Design review of the part built by this model. Coordinates are the model's own, in mm. A direction names the side the tool comes from. Coordinates: 2 decimals unless noted, no trailing zeros. Write each loop counter-clockwise with the first axis right and the second up, starting at its lowest first coordinate (ties: lowest second). Pieces come first, ordered by that corner, then holes.
```python
from build123d import *

# Parameters (mm, degrees)
SKETCH1_W           = 7
SKETCH1_H           = 7
BOSS_EXTRUDE1_DEPTH = 5
SKETCH4_R           = 1.65
CUT_EXTRUDE4_DEPTH  = 4
SKETCH6_R           = 1.65
CUT_EXTRUDE6_DEPTH  = 4
SKETCH6_4_R         = 1.65
BOSS_EXTRUDE2_DEPTH = 1.48


with BuildPart() as part:
    # Sketch1 → Boss-Extrude1 (new body)
    with BuildSketch(Plane(origin=(0, 0, 0), x_dir=(1, 0, 0), z_dir=(0, 1, 0))):
        with Locations((-0.67779661, -2.128287226)):
            Rectangle(SKETCH1_W, SKETCH1_H)
    extrude(amount=BOSS_EXTRUDE1_DEPTH)

    # Sketch4 → Cut-Extrude4 (cut)
    with BuildSketch(Plane(origin=(0, 5, 0), x_dir=(1, 0, 0), z_dir=(0, 1, 0))):
        Polygon((-1.544486233, 1.106242481), (-3.912326317, -1.261597603), (-3.045636694, -4.496127311), (0.188893013, -5.362816934), (2.556733098, -2.99497685), (1.690043475, 0.239552858), align=None)
        with Locations((-0.67779661, -2.128287226)):
            Circle(SKETCH4_R, mode=Mode.SUBTRACT)
    extrude(amount=-CUT_EXTRUDE4_DEPTH, mode=Mode.SUBTRACT)

    # Sketch6 → Cut-Extrude6 (cut)
    with BuildSketch(Plane(origin=(0, 5, 0), x_dir=(1, 0, 0), z_dir=(0, 1, 0))):
        with Locations((-0.67779661, -2.128287226)):
            Circle(SKETCH6_R)
    extrude(amount=-CUT_EXTRUDE6_DEPTH, mode=Mode.SUBTRACT)

    # Sketch6_4 → Boss-Extrude2 (add)
    with BuildSketch(Plane(origin=(0, 5, 0), x_dir=(1, 0, 0), z_dir=(0, 1, 0))):
        Polygon((1.690043475, 0.239552858), (-1.544486233, 1.106242481), (-3.912326317, -1.261597603), (-3.045636694, -4.496127311), (0.188893013, -5.362816934), (2.556733098, -2.99497685), align=None)
        with Locations((-0.67779661, -2.128287226)):
            Circle(SKETCH6_4_R, mode=Mode.SUBTRACT)
    extrude(amount=-BOSS_EXTRUDE2_DEPTH)


solid = part.part
```
(1) Mouldability with a two-part tool opening along X and no side actions: class faces 1 (the flat face through (-3.485, 2.278, 2.856)), 2 (the flat face through (2.822, 2, 2)), 3 (the flat face through (-1, 2, 5.628)) as +X half, -X half, draft (parallel to the pull), parting line (faces both ways), or undercut.
(2) For faces 4 (the flat face through (-1, 2, -1.372)), 5 (the flat face through (-2.2, 3.52, 0.6)), 6 (the cylindrical face through (-0.89, 4.27, 0.49)), list the 3-axis set-ups (+Z, -Z, +X, -X, +Y, -Y) from which the entire face can be reached by the end or side of a thin tool; tool diameter is ignored.
(3) Consider section A-A (y = 2.6). Give the boundary of the cut face in (x, z).
(4) Wall thickness on line 1 (Y direction, x = 0.5, z = 0); line 2 (X direction, y = 3.2, z = 0.25); line 3 (Z direction, x = -3, y = 2.1): over which ranges is each line inside the solid? List them lowest first.
(5) Consider section B-B (z = -0.5). Give the boundary of the cut face in (x, y).
(6) Consider section C-C (x = 1.25). Give the boundary of the cut face in (y, z).
(7) Consider section D-D (z = 0.75). Give the boundary of the cut face in (x, y), plus the area to 3 significant figures.
Results:
1. face 1: undercut
1. face 2: +X half
1. face 3: draft
2. face 4: -Z, +X, -X, +Y, -Y
2. face 5: none
2. face 6: +Y
3. outline: (-4.18, -1.37) - (2.82, -1.37) - (2.82, 5.63) - (-4.18, 5.63) - close; hole (-3.91, 1.26) - (-1.54, -1.11) - (1.69, -0.24) - (2.56, 2.99) - (0.19, 5.36) - (-3.05, 4.5) - close
4. line 1: y = 0 to 1, 3.52 to 5
4. line 2: x = -4.18 to -2.9, 1.82 to 2.82
4. line 3: z = -1.37 to 0.35, 4.51 to 5.63
5. outline: (-4.18, 0) - (2.82, 0) - (2.82, 5) - (-4.18, 5) - close; hole (-2.15, 1) - (0.72, 1) - (0.72, 3.52) - (-2.15, 3.52) - close
6. outline: (0, -1.37) - (5, -1.37) - (5, 5.63) - (0, 5.63) - close; hole (1, -0.36) - (3.52, -0.36) - (3.52, 4.3) - (1, 4.3) - close
7. outline: (-4.18, 0) - (2.82, 0) - (2.82, 5) - (0.23, 5) - (0.23, 3.52) - (1.96, 3.52) - (1.96, 1) - (-3.4, 1) - (-3.4, 3.52) - (-1.58, 3.52) - (-1.58, 5) - (-4.18, 5) - close
7. area: 18.8 mm2
